Geometry check sheet. Reference: the model listing, model coordinates, mm. Face numbers are marked on the shaded views. Round coordinates to 2 decimals unless told otherwise and drop trailing zeros. Order: outer loops, then holes, each group sorted by start corner. A loop starts at its lowest first (then second) coordinate and runs counter-clockwise, first axis right, second up. Notation, with made-up numbers: (-23, 67) -> (28, 67) arc R19 cw to (28, 99) -> close; hole circle Ø6 at (-24.75, 29). An arc over 180 degrees is marked (long way). Answer as a JSON object with one key per item and string values. Group by question number.
from build123d import *

# Parameters (mm, degrees)
SKETCH_1_W          = 156.75
SKETCH_1_H          = 105.271994628
EXTRUDE_1_DEPTH     = 12.2
SKETCH_2_W          = 7.639581741
SKETCH_2_H          = 13.89014237
CUT_EXTRUDE_1_DEPTH = 6.1
SKETCH_4_R          = 5.5
EXTRUDE_2_DEPTH     = 18
EXTRUDE_2_TAPER     = 5
CUT_EXTRUDE_2_REACH = 20
SKETCH_6_R          = 1.55
SKETCH_7_W          = 7
SKETCH_7_H          = 3.5
CUT_EXTRUDE_3_DEPTH = 9.1


with BuildPart() as part:
    # ｽｹｯﾁ1 → ﾎﾞｽ - 押し出し1 (new body)
    with BuildSketch(Plane(origin=(0, 0, 0), x_dir=(1, 0, 0), z_dir=(0, 1, 0))):
        Rectangle(SKETCH_1_W, SKETCH_1_H)
    extrude(amount=EXTRUDE_1_DEPTH)

    # ｽｹｯﾁ2 → ｶｯﾄ - 押し出し1 (cut)
    with BuildSketch(Plane(origin=(0, 12.2, 0), x_dir=(1, 0, 0), z_dir=(0, 1, 0))):
        with BuildLine():
            ThreePointArc((-44.016, 13.890145056), (-40.196209129, 16.500447871), (-36.376418259, 13.890145056))
            Line((-36.376418259, 13.890145056), (-44.016, 13.890145056))
        make_face()
        with Locations((-40.19620913, 6.945073871)):
            Rectangle(SKETCH_2_W, SKETCH_2_H)
        with BuildLine():
            Line((-44.016, 2.686e-06), (-36.376418259, 2.686e-06))
            ThreePointArc((-36.376418259, 2.686e-06), (-40.196209129, -2.610300128), (-44.016, 2.686e-06))
        make_face()
        with BuildLine():
            Line((44.016, 13.890145056), (36.376418259, 13.890145056))
            ThreePointArc((36.376418259, 13.890145056), (40.196209129, 16.500447871), (44.016, 13.890145056))
        make_face()
        with Locations((40.19620913, 6.945073871)):
            Rectangle(SKETCH_2_W, SKETCH_2_H)
        with BuildLine():
            ThreePointArc((44.016, 2.686e-06), (40.196209129, -2.610300128), (36.376418259, 2.686e-06))
            Line((36.376418259, 2.686e-06), (44.016, 2.686e-06))
        make_face()
    extrude(amount=-CUT_EXTRUDE_1_DEPTH, mode=Mode.SUBTRACT)

    # ｽｹｯﾁ4 → ﾎﾞｽ - 押し出し2 (add)
    with BuildSketch(Plane.XY.offset(52.635997314)):
        with Locations((-22.875, 6.1)):
            Circle(SKETCH_4_R)
        with Locations((22.875, 6.1)):
            Circle(SKETCH_4_R)
    extrude(amount=EXTRUDE_2_DEPTH, taper=EXTRUDE_2_TAPER)

    # ｽｹｯﾁ6 → ｶｯﾄ - 押し出し2 (cut, up to next)
    with BuildSketch(Plane.XY.offset(52.635997314), mode=Mode.PRIVATE) as cut_extrude_2_sk1:
        with Locations((-22.875, 6.1)):
            Circle(SKETCH_6_R)
    cut_extrude_2_tool1 = extrude(cut_extrude_2_sk1.sketch, amount=CUT_EXTRUDE_2_REACH, mode=Mode.PRIVATE) & part.part
    add(cut_extrude_2_tool1.solids().sort_by_distance((-22.875, 6.1, 52.635997))[0], mode=Mode.SUBTRACT)
    # ｽｹｯﾁ6 → ｶｯﾄ - 押し出し2 (cut, up to next)
    with BuildSketch(Plane.XY.offset(52.635997314), mode=Mode.PRIVATE) as cut_extrude_2_sk2:
        with Locations((22.875, 6.1)):
            Circle(SKETCH_6_R)
    cut_extrude_2_tool2 = extrude(cut_extrude_2_sk2.sketch, amount=CUT_EXTRUDE_2_REACH, mode=Mode.PRIVATE) & part.part
    add(cut_extrude_2_tool2.solids().sort_by_distance((22.875, 6.1, 52.635997))[0], mode=Mode.SUBTRACT)

    # ｽｹｯﾁ7 → ｶｯﾄ - 押し出し3 (cut)
    with BuildSketch(Plane(origin=(0, 0, 0), x_dir=(1, 0, 0), z_dir=(0, 1, 0))):
        with Locations((-22.875, -58.885997314)):
            Rectangle(SKETCH_7_W, SKETCH_7_H)
        with Locations((22.875, -58.885997314)):
            Rectangle(SKETCH_7_W, SKETCH_7_H)
    extrude(amount=CUT_EXTRUDE_3_DEPTH, mode=Mode.SUBTRACT)


solid = part.part
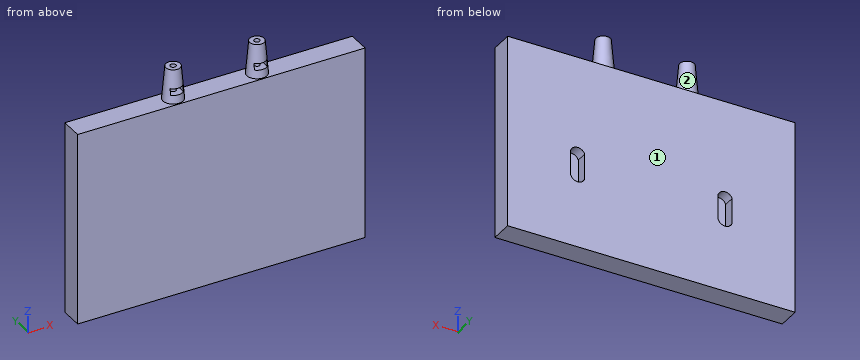
Item 1: Sectioned sample at B-B, the plane x = -49.5. Enter the section's corners in (y, z), then the cut area to 3 significant figures.
Item 2: Sectioned sample at A-A, the plane z = -3.5. Enter the section's corners in (x, y) (3 decimals).
Item 3: Mould release check, pull along X, two halves, no side actions. Record for the marked faces 1 and 2: pulls with the +X half, pulls with the -X half, needs draft (parallel to the pull), parting line crosses it, or undercut.
Item 4: Depth check by flat-ended pin: pin 1 Ø1.5 at (x, y) = (-22.5, 5.5) entering from +Z; pin 2 Ø3 at (y, z) = (5, 58.5) entering from +X; pin 3 Ø4 at (x, z) = (24, 59) entering from -Y; pin 4 Ø4 at (x, y) = (-22.875, 6.1) entering from +Z. Enter the tip coordinate at first touch or a pass-through.
Item 5: Thickness scan on L1, parallel to X at y = 6.1, z = 65.25 (3 decimals); L2, parallel to X at y = 6.1, z = 64 (3 decimals); L3, parallel to Z at x = 70.5, y = 1.75. Record the ranges inside material, lowest first.
Result:
{
 "1": {"outline": "(0, -52.64) -> (12.2, -52.64) -> (12.2, 52.64) -> (0, 52.64) -> close", "area": "1,280 mm2"},
 "2": {"outline": "(-78.375, 0) -> (78.375, 0) -> (78.375, 12.2) -> (44.016, 12.2) -> (44.016, 6.1) -> (36.376, 6.1) -> (36.376, 12.2) -> (-36.376, 12.2) -> (-36.376, 6.1) -> (-44.016, 6.1) -> (-44.016, 12.2) -> (-78.375, 12.2) -> close"},
 "3": {"face 1": "needs draft", "face 2": "undercut"},
 "4": {"pin 1": "stops at z = 52.64", "pin 2": "stops at x = 27.96", "pin 3": "stops at y = 1.01", "pin 4": "stops at z = 70.64"},
 "5": {"L1": "x = -27.271 to -24.425, -21.325 to -18.479, 18.479 to 21.325, 24.425 to 27.271", "L2": "x = -27.381 to -24.425, -21.325 to -18.369, 18.369 to 21.325, 24.425 to 27.381", "L3": "z = -52.64 to 52.64"}
}
